Here's how the part is built. I have some questions about the finished solid (model axes, mm). A direction names the side the tool comes from. Round coordinates to 2 decimals unless told otherwise and drop trailing zeros. Loops run counter-clockwise (first coordinate to the right, second up) from the corner with the lowest first, then second, coordinate; pieces in that order, holes last. Notation, with made-up numbers: M 44.5,-33 L 94.5,-33 A12 ccw 94.5,-16 Z; hole C -34.5,10 d8. An arc over 180 degrees is marked long. Use a Markdown table: item, result.
```python
from build123d import *

# Parameters (mm, degrees)
F0_W      = 111.3092452288
F0_H      = 110.8992248774
F1_DEPTH  = 100.076
F2_R      = 19.073919737
F2_R_2    = 19.3546495163
F3_DEPTH  = 51.816
F4_R      = 12.7
F4_R_2    = 6.35
F5_DEPTH  = 2.54
F6_DEPTH  = 5.08
F8_DEPTH  = 2.54
F10_R     = 14.0521867963
F11_DEPTH = 20.066
F12_R     = 16.1662209707
F13_DEPTH = 23.368
F14_R     = 12.7
F15_DEPTH = 25.4


with BuildPart() as f1:
    # F0 (on Front) → F1 (new body)
    with BuildSketch(Plane.XZ):
        Rectangle(F0_W, F0_H)
    extrude(amount=F1_DEPTH)

    # F2 (on face) → F3 (join)
    with BuildSketch(Plane.XY.offset(55.4496124387)):
        with Locations((-35.2833792567, -42.3366203904)):
            Circle(F2_R)
        with Locations((31.1419349164, -48.2057631016)):
            Circle(F2_R_2)
    extrude(amount=F3_DEPTH)

    # F4 (on face) → F5 (join)
    with BuildSketch(Plane.XZ.offset(100.076)):
        with Locations((-29.463622719, 25.3433045)):
            Circle(F4_R)
        with Locations((-29.463622719, 25.3433045)):
            Circle(F4_R_2, mode=Mode.SUBTRACT)
        with Locations((30.5558927357, 25.3433045)):
            Circle(F4_R)
        with Locations((30.5558927357, 25.3433045)):
            Circle(F4_R_2, mode=Mode.SUBTRACT)
    extrude(amount=F5_DEPTH)

    # F6 (add): faces of the model
    f6_faces = [f1.faces().sort_by_distance(p)[0] for p in [
        (-29.463622719, -100.076, 25.3433045),
        (30.5558927357, -100.076, 25.3433045),
    ]]
    extrude(f6_faces, amount=F6_DEPTH)

    # F7 (on face) → F8 (join)
    with BuildSketch(Plane.XZ.offset(100.076)):
        with BuildLine():
            add(Edge.make_bspline(
                [(-15.1932500303, -14.5297981799), (-11.5570264912, -7.3093204863), (28.4939557063, -6.8955534703), (4.9116646059, -45.832072352), (-18.5883527484, -21.2714803619), (-15.1932500303, -14.5297981799)],
                knots=[0, 0, 0, 0, 0.3589682542, 0.6648352109, 1, 1, 1, 1], degree=3))
        make_face()
    extrude(amount=F8_DEPTH)

    # F10 (on face) → F11 (join)
    with BuildSketch(Plane(origin=(-55.6546226144, 0, 0), x_dir=(0, -1, 0), z_dir=(-1, 0, 0))):
        with Locations((48.5344566405, 0)):
            Circle(F10_R)
    extrude(amount=F11_DEPTH)

    # F12 (on face) → F13 (join)
    with BuildSketch(Plane.YZ.offset(55.6546226144)):
        with Locations((-48.6368350685, 0)):
            Circle(F12_R)
    extrude(amount=F13_DEPTH)

    # F14 (on face) → F15 (join)
    with BuildSketch(Plane(origin=(0, 0, -55.4496124387), x_dir=(1, 0, 0), z_dir=(0, 0, -1))):
        with Locations((-22.938253358, 52.1185323596)):
            Circle(F14_R)
        with Locations((25.9563419968, 52.1185323596)):
            Circle(F14_R)
    extrude(amount=F15_DEPTH)


solid = f1.part
```
Q1. Imagine slicing it at B-B, the plane y = -83. Please give me the cut outline in (x, z).
Return value:
| item | result |
|---|---|
| outline | M -55.65,-55.45 L 55.65,-55.45 L 55.65,55.45 L -55.65,55.45 Z |
Q2. We'd pull the mould along X, two halves only. Please class faces 1 (the flat face through (-36, -42, 107.266)), 2 (the flat face through (79.023, -49, 0)), 3 (the cylindrical face through (-25.69, -39.72, -67.97)): pulls with the +X half, pulls with the -X half, needs draft (parallel to the pull), parting line crosses it, or undercut.
Return value:
| item | result |
|---|---|
| face 1 | needs draft |
| face 2 | pulls with the +X half |
| face 3 | undercut |
Q3. For faces 4 (the flat face through (-1, -100.076, 1)), 5 (the flat face through (-1, -49, 55.45)), 6 (the flat face through (-55.655, -60, -13)), 7 (the flat face through (-75.721, -48, 0)), 8 (the cylindrical face through (67.18, -60.55, 10.93)), which set-ups out of +Z, -Z, +X, -X, +Y, -Y let a thin tool reach every point of the face, with its end or its side?
Return value:
| item | result |
|---|---|
| face 4 | -Y |
| face 5 | +Z |
| face 6 | -X |
| face 7 | +Z, -Z, -X, +Y, -Y |
| face 8 | +X |
Q4. Imagine slicing it at A-A, the plane z = 0. Please give me the cut outline in (x, y).
Return value:
| item | result |
|---|---|
| outline | M -75.72,-62.59 L -55.65,-62.59 L -55.65,-100.08 L 55.65,-100.08 L 55.65,-64.8 L 79.02,-64.8 L 79.02,-32.47 L 55.65,-32.47 L 55.65,0 L -55.65,0 L -55.65,-34.48 L -75.72,-34.48 Z |
Q5. Will these pins go through, and if not, where does the flat tip stop? P1, Ø2, axis at x = 27.5, z = -55, coming from the -Y side; P2, Ø1, axis at x = 25.5, z = 66, coming from the -Y side; P3, Ø12, axis at x = -0.5, y = -65.5, coming from the +Z side.
Return value:
| item | result |
|---|---|
| P1 | stops at y = -100.08 |
| P2 | stops at y = -66.86 |
| P3 | stops at z = 55.45 |
Q6. I need wall thicknesses on line 1 (Y direction, x = -11.5, z = 36.5); line 2 (Z direction, x = 34, y = -27); line 3 (X direction, y = -25.5, z = -15). Which ranges of each line are inside material? Lowest first, please. Write a range as from..to.
Return value:
| item | result |
|---|---|
| line 1 | y = -100.08..0 |
| line 2 | z = -55.45..55.45 |
| line 3 | x = -55.65..55.65 |
Q7. Imagine slicing it at C-C, the plane z = -67.5. Please give me the cut outline in (x, y), then the cut area to 3 significant figures.
Return value:
| item | result |
|---|---|
| outline | C -22.94,-52.12 d25.4; C 25.96,-52.12 d25.4 |
| area | 1,010 mm^2 |
Q8. Imagine slicing it at D-D, the plane x = -49. Please give me the cut outline in (y, z).
Return value:
| item | result |
|---|---|
| outline | M -100.08,-55.45 L 0,-55.45 L 0,55.45 L -29.08,55.45 L -29.08,107.27 L -55.59,107.27 L -55.59,55.45 L -100.08,55.45 Z |
